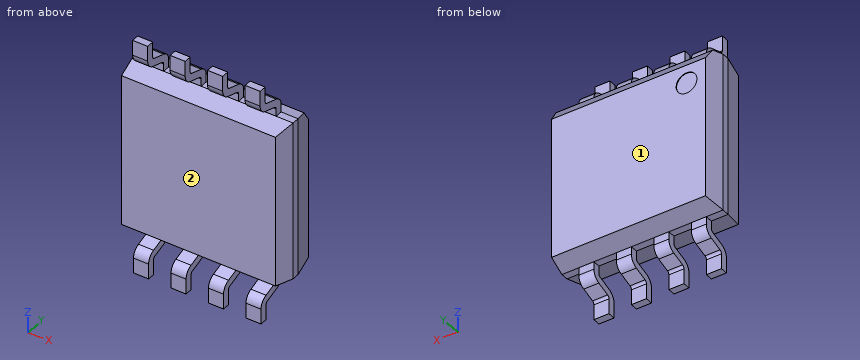
```python
from build123d import *

# Parameters (mm, degrees)
BOSS_EXTRUDE1_DEPTH      = 0.125
BOSS_EXTRUDE1_DEPTH_BACK = 0.125
SKETCH1_W                = 5.46
SKETCH1_H                = 5.41
SKETCH2_W                = 5.46
SKETCH2_H                = 5.41
BOSS_EXTRUDE2_DEPTH      = 0.7
BOSS_EXTRUDE2_TAPER      = 10
SKETCH3_W                = 5.46
SKETCH3_H                = 5.41
BOSS_EXTRUDE3_DEPTH      = 0.7
BOSS_EXTRUDE3_TAPER      = 10
CHAMFER1_SIZE            = 0.3
CHAMFER1_SIZE2           = 0.369840916
BOSS_EXTRUDE4_START      = 0.3775
BOSS_EXTRUDE4_DEPTH      = 0.51
LPATTERN1_COUNT          = 2
LPATTERN1_PITCH          = 1.27
LPATTERN1_COL_COUNT      = 3
LPATTERN1_COL_PITCH      = 1.27
SKETCH6_R                = 0.351785146
CUT_EXTRUDE1_DEPTH       = 0.02


with BuildPart() as part:
    # Sketch1 → Boss-Extrude1 (new, two sides: drawn at the far end of the back side and taken through both)
    with BuildSketch(Plane(origin=(0, 0.92, 0), x_dir=(1, 0, 0), z_dir=(0, 1, 0)).offset(-BOSS_EXTRUDE1_DEPTH_BACK)):
        Rectangle(SKETCH1_W, SKETCH1_H)
    extrude(amount=BOSS_EXTRUDE1_DEPTH + BOSS_EXTRUDE1_DEPTH_BACK)

    # Sketch2 → Boss-Extrude2 (add)
    with BuildSketch(Plane(origin=(0, 1.045, 0), x_dir=(1, 0, 0), z_dir=(0, 1, 0))):
        Rectangle(SKETCH2_W, SKETCH2_H)
    extrude(amount=BOSS_EXTRUDE2_DEPTH, taper=BOSS_EXTRUDE2_TAPER)

    # Sketch3 → Boss-Extrude3 (add)
    with BuildSketch(Plane.XZ.offset(-0.795)):
        Rectangle(SKETCH3_W, SKETCH3_H)
    extrude(amount=BOSS_EXTRUDE3_DEPTH, taper=BOSS_EXTRUDE3_TAPER)

    # Chamfer1
    chamfer1_edges = [part.edges().sort_by_distance(p)[0] for p in [
        (0, 1.745, 2.581571114),
    ]]
    chamfer1_side = [part.faces().sort_by_distance(p)[0] for p in [
        (0, 1.392301631, 2.643761352),
    ]]
    chamfer(chamfer1_edges, length=CHAMFER1_SIZE, length2=CHAMFER1_SIZE2, reference=chamfer1_side[0])

    # Sketch5 → Boss-Extrude4 (add)
    with BuildSketch(Plane(origin=(0, 0, 0), x_dir=(0, 0, -1), z_dir=(1, 0, 0)).offset(BOSS_EXTRUDE4_START)):
        with BuildLine():
            ThreePointArc((-3.20280312, 0.243081155), (-3.329274491, 0.063778027), (-3.537635241, -0.005))
            Line((-3.537635241, -0.005), (-4.051646267, -0.005))
            Line((-4.051646267, -0.005), (-4.051646267, 0.245))
            Line((-4.051646267, 0.245), (-3.537635241, 0.245))
            ThreePointArc((-3.537635241, 0.245), (-3.478103598, 0.264650865), (-3.441968921, 0.31588033))
            Line((-3.441968921, 0.31588033), (-3.295422291, 0.796918845))
            ThreePointArc((-3.295422291, 0.796918845), (-3.168950919, 0.976221974), (-2.960590167, 1.045000002))
            Line((-2.960590167, 1.045000002), (-2.704999997, 1.045000002))
            Line((-2.704999997, 1.045000002), (-2.704999997, 0.794999999))
            Line((-2.704999997, 0.794999999), (-2.960590167, 0.794999999))
            ThreePointArc((-2.960590167, 0.794999999), (-3.020112307, 0.775356174), (-3.056249597, 0.724142296))
            Line((-3.056249597, 0.724142296), (-3.20280312, 0.243081155))
        make_face()
        with BuildLine():
            Line((2.704999997, 0.794999999), (2.960590167, 0.794999999))
            ThreePointArc((2.960590167, 0.794999999), (3.020112307, 0.775356174), (3.056249597, 0.724142296))
            Line((3.056249597, 0.724142296), (3.201156853, 0.288081155))
            ThreePointArc((3.201156853, 0.288081155), (3.327628224, 0.108778027), (3.535988974, 0.04))
            Line((3.535988974, 0.04), (4.05, 0.04))
            Line((4.05, 0.04), (4.05, 0.29))
            Line((4.05, 0.29), (3.535988974, 0.29))
            ThreePointArc((3.535988974, 0.29), (3.476457331, 0.309650865), (3.440322653, 0.36088033))
            Line((3.440322653, 0.36088033), (3.295422291, 0.796918845))
            ThreePointArc((3.295422291, 0.796918845), (3.168950919, 0.976221974), (2.960590167, 1.045000002))
            Line((2.960590167, 1.045000002), (2.704999997, 1.045000002))
            Line((2.704999997, 1.045000002), (2.704999997, 0.794999999))
        make_face()
    boss_extrude4 = extrude(amount=BOSS_EXTRUDE4_DEPTH)

    # LPattern1: Boss-Extrude4 ×2
    with Locations(*[(i * LPATTERN1_PITCH, 0, 0) for i in range(1, LPATTERN1_COUNT)]):
        add(boss_extrude4)

    # LPattern1 col: Boss-Extrude4 ×3
    with Locations(*[(-i * LPATTERN1_COL_PITCH, 0, 0) for i in range(1, LPATTERN1_COL_COUNT)]):
        add(boss_extrude4)

    # Sketch6 → Cut-Extrude1 (cut)
    with BuildSketch(Plane(origin=(0, 1.745, 0), x_dir=(1, 0, 0), z_dir=(0, 1, 0))):
        with Locations(Location((-1.967714846, -1.59473048, 0), (0, 0, 270))):
            Circle(SKETCH6_R)
    extrude(amount=-CUT_EXTRUDE1_DEPTH, mode=Mode.SUBTRACT)


solid = part.part
```
The listing builds one solid part. Answer for the finished solid, in the listing's coordinates (mm). Face numbers are marked on the shaded views. Round coordinates to 2 decimals unless told otherwise and drop trailing zeros.
Q1. For a pull along Z with two mould halves and no side action, classify the marked faces 1 and 2 as released by +Z, released by -Z, zero draft, split by the parting line, or undercut.
Q2. Find the intervals of material crossed by line 1 (X direction, y = 0.9, z = -3); line 2 (Y direction, x = 2.1, z = 0.5) (3 decimals); line 3 (X direction, y = 1.45, z = 1.75), in increasing order.
Q3. Section A-A, the plane y = 0.5 is taken. Count the separate pieces of the cut face and the enclosed holes in it, then the cut area to 3 significant figures.
Q4. Given pin 1 Ø0.8 at (y, z) = (0.5, -3.5) entering from -X; pin 2 Ø0.5 at (y, z) = (0.5, -3.5) entering from +X, each flat-ended and moving along its own axis, determine where each tip first touches the part or whether it passes through.
Completed:
1. face 1: zero draft
1. face 2: undercut
2. line 1: x = -2.16 to -1.65, -0.89 to -0.38, 0.38 to 0.89, 1.65 to 2.16
2. line 2: y = 0.095 to 1.745
2. line 3: x = -2.66 to 2.66
3. separate pieces: 9
3. enclosed holes: 0
3. area: 29.5 mm2
4. pin 1: stops at x = -2.16
4. pin 2: stops at x = 2.16
